from build123d import *

# Parameters (mm, degrees)
F0_W     = 25.4
F0_H     = 47.049225
F1_DEPTH = 12.7
F2_W     = 17.78
F2_H     = 17.78
F3_DEPTH = 240.03
F4_R     = 1.893959
F5_DEPTH = 63.5
F6_R     = 5.08


with BuildPart() as f1:
    # F0 (on Front) → F1 (new body, symmetric)
    with BuildSketch(Plane.XZ):
        with Locations((2.46951, 16.322443)):
            Rectangle(F0_W, F0_H)
        Polygon((-61.03049, -7.202169), (-61.03049, -32.602169), (65.96951, -32.602169), (65.96951, -7.202169), (15.16951, -7.202169), (-10.23049, -7.202169), align=None)
    extrude(amount=F1_DEPTH, both=True)

    # F2 (on face) → F3 (cut, symmetric)
    with BuildSketch(Plane.YZ.offset(65.96951)):
        with Locations((0, -19.902169)):
            Rectangle(F2_W, F2_H)
    extrude(amount=F3_DEPTH, both=True, mode=Mode.SUBTRACT)

    # F4 (on face) → F5 (cut, symmetric)
    with BuildSketch(Plane.XY.offset(39.847056)):
        with Locations((2.532323, 0)):
            Circle(F4_R)
    extrude(amount=-F5_DEPTH, both=True, mode=Mode.SUBTRACT)

    # F6
    f6_edges = [f1.edges().sort_by_distance(p)[0] for p in [
        (40.56951, -12.7, -7.202169),
        (40.56951, 12.7, -7.202169),
        (-35.63049, -12.7, -7.202169),
        (-35.63049, 12.7, -7.202169),
        (2.46951, -12.7, -32.602169),
        (2.46951, 12.7, -32.602169),
        (15.16951, -12.7, 16.322444),
        (-10.23049, -12.7, 16.322444),
        (-10.23049, 12.7, 16.322444),
        (15.16951, 12.7, 16.322444),
        (2.46951, 12.7, 39.847056),
        (15.16951, 0, 39.847056),
        (2.46951, -12.7, 39.847056),
        (-10.23049, 0, 39.847056),
    ]]
    fillet(f6_edges, radius=F6_R)


solid = f1.part
Can you work these out from the model? Positions are in its coordinate system, mm. A direction names the side the tool comes from. Coordinates: 2 decimals unless noted, no trailing zeros. Write each loop counter-clockwise with the first axis right and the second up, starting at its lowest first coordinate (ties: lowest second). Pieces come first, ordered by that corner, then holes.
Q1. Imagine slicing it at B-B, the plane z = -17.5. List the corners of the cut face in (x, y) for me.
Results found:
outline: (-61.03, -12.7) - (65.97, -12.7) - (65.97, -8.89) - (-61.03, -8.89) - close; (-61.03, 8.89) - (65.97, 8.89) - (65.97, 12.7) - (-61.03, 12.7) - close
Q2. If we mould it in two halves opening along Z, with no side actions, what happens to faces 1 (the face through (0.64, 0.08, 14.77)), 2 (the face through (-8.8, 0.1, 38.3)), 3 (the face through (3, 0, -28.792))? For each: +Z half, -Z half, draft (parallel to the pull), parting line (faces both ways), or undercut.
Results found:
face 1: draft
face 2: +Z half
face 3: undercut
Q3. Imagine slicing it at C-C, the plane x = -20. List the corners of the cut face in (y, z) for me.
Results found:
outline: (-12.7, -27.52) arc R5.08 ccw to (-7.62, -32.6) - (7.62, -32.6) arc R5.08 ccw to (12.7, -27.52) - (12.7, -12.28) arc R5.08 ccw to (7.62, -7.2) - (-7.62, -7.2) arc R5.08 ccw to (-12.7, -12.28) - close; hole (-8.89, -28.79) - (8.89, -28.79) - (8.89, -11.01) - (-8.89, -11.01) - close
Q4. Please list where these lines run through material, in increasing order: L1, parallel to Z at x = 44, y = 7.25; L2, parallel to Z at x = -0.5, y = 7.5; L3, parallel to Y at x = -6, z = -28.
Results found:
L1: z = -32.6 to -28.79, -11.01 to -7.2
L2: z = -32.6 to -28.79, -11.01 to 39.85
L3: y = -12.68 to -8.89, 8.89 to 12.68
Q5. Imagine slicing it at D-D, the plane z = 23.5. List the corners of the cut face in (x, y) for me.
Results found:
outline: (-10.23, -7.62) arc R5.08 ccw to (-5.15, -12.7) - (10.09, -12.7) arc R5.08 ccw to (15.17, -7.62) - (15.17, 7.62) arc R5.08 ccw to (10.09, 12.7) - (-5.15, 12.7) arc R5.08 ccw to (-10.23, 7.62) - close; hole circle Ø3.79 at (2.53, 0)
Q6. Imagine slicing it at A-A, the plane y = -3.5. List the corners of the cut face in (x, z) for me, plus the area to 3 significant figures.
Results found:
outline: (-61.03, -32.6) - (65.97, -32.6) - (65.97, -28.79) - (-61.03, -28.79) - close; (-61.03, -11.01) - (65.97, -11.01) - (65.97, -7.2) - (15.17, -7.2) - (15.17, 34.77) arc R5.08 ccw to (10.09, 39.85) - (-5.15, 39.85) arc R5.08 ccw to (-10.23, 34.77) - (-10.23, -7.2) - (-61.03, -7.2) - close
area: 2,150 mm2
Q7. Which directions (+Z, -Z, +X, -X, +Y, -Y) give clear straight access to the entire face, cutting with the end or side of a thin tool? Please do faces 4 (the face through (-8.703, 11.251, 11.572)), 5 (the face through (-10.23, 0, 13)), 6 (the face through (37.64, 11.25, -8.73)), 7 (the face through (41, 0, -7.202)).
Results found:
face 4: +Z, -X, +Y
face 5: +Z, -X, +Y, -Y
face 6: +Z, +X, +Y
face 7: +Z, +X, +Y, -Y
Q8. For P1, Ø4.5, axis at y = -3, z = 5.5, coming from the +X side; P2, Ø4.5, axis at x = -38, y = 0, coming from the +Z side; P3, Ø4.5, axis at y = 0, z = 18, coming from the -X side, each with a flat end and sliding along its axis, tell me the tip position at first contact or that it passes through.
Results found:
P1: stops at x = 15.17
P2: stops at z = -7.2
P3: stops at x = -10.23
